Verification items for this drawing (mm, ordinates from the low corner). A direction names the side the tool comes from. Coordinates: 2 decimals unless noted, no trailing zeros. Write each loop counter-clockwise with the first axis right and the second up, starting at its lowest first coordinate (ties: lowest second). Pieces come first, ordered by that corner, then holes. Notation, with made-up numbers: (-11.75, -36) -> (-0.75, -36) arc R28 cw to (-0.75, -8) -> close; hole circle Ø4 at (-29, 47). An arc over 180 degrees is marked (long way). One line per question, with ' | ' between items.
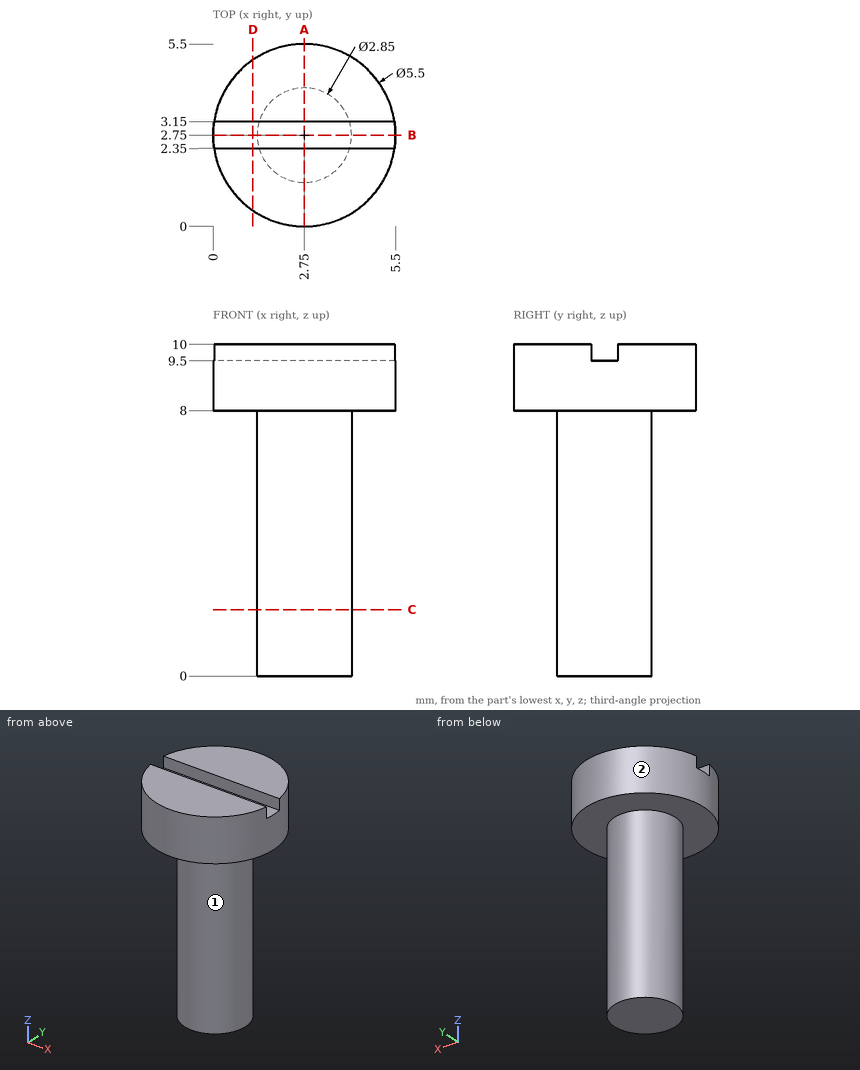
(1) Material ranges on line 1 (Z direction, x = 3.15, y = 1.1); line 2 (Y direction, x = 2.7, z = 7.5); line 3 (Z direction, x = 1.25, y = 2.6), recorded low to high.
Answers below:
line 1: z = 8 to 10 | line 2: y = 1.33 to 4.17 | line 3: z = 8 to 9.5
(2) Cross-section at D-D (x = 1.2). Record the cut outline in (y, z).
Answers below:
outline: (0.48, 8) -> (5.02, 8) -> (5.02, 10) -> (3.15, 10) -> (3.15, 9.5) -> (2.35, 9.5) -> (2.35, 10) -> (0.48, 10) -> close
(3) Depth check by flat-ended pin: P1, Ø1, axis at x = 2, y = 3, coming from the -Z side. Enter the tip coordinate at first touch or a pass-through.
Answers below:
P1: stops at z = 0
(4) Tool access check on the marked faces 1 and 2. Record the directions out of +Z, -Z, +X, -X, +Y, -Y that give a thin tool (end or side, any length) a straight path to the whole face; none if there is none.
Answers below:
face 1: -Z | face 2: +Z, -Z
(5) Cross-section at A-A (x = 2.75). Record the cut outline in (y, z) (3 decimals), plus the area to 3 significant figures.
Answers below:
outline: (0, 8) -> (1.325, 8) -> (1.325, 0) -> (4.175, 0) -> (4.175, 8) -> (5.5, 8) -> (5.5, 10) -> (3.15, 10) -> (3.15, 9.5) -> (2.35, 9.5) -> (2.35, 10) -> (0, 10) -> close | area: 33.4 mm²
(6) Cross-section at C-C (z = 2). Record the cut outline in (x, y) (3 decimals), plus the area to 3 significant figures.
Answers below:
outline: circle Ø2.85 at (2.75, 2.75) | area: 6.38 mm²
(7) Cross-section at B-B (y = 2.75). Record the cut outline in (x, z) (3 decimals).
Answers below:
outline: (0, 8) -> (1.325, 8) -> (1.325, 0) -> (4.175, 0) -> (4.175, 8) -> (5.5, 8) -> (5.5, 9.5) -> (0, 9.5) -> close
